Here's how the part is built. I have some questions about the finished solid (model axes, mm). Round coordinates to 2 decimals unless told otherwise and drop trailing zeros. Write each loop counter-clockwise with the first axis right and the second up, starting at its lowest first coordinate (ties: lowest second). Pieces come first, ordered by that corner, then holes. Notation, with made-up numbers: (-35, -33) -> (-3, -33) arc R21 cw to (-3, 1) -> close; hole circle Ø5 at (22, 30). An arc over 180 degrees is marked (long way). Answer in a Markdown table with one row per item.
from build123d import *

# Parameters (mm, degrees)
F0_W     = 457.2
F0_H     = 50.8
F1_DEPTH = 101.6
F2_W     = 98.554954
F2_H     = 50.8
F3_DEPTH = 2438.4
F4_W     = 457.2
F4_H     = 101.6
F5_DEPTH = 50.8


with BuildPart() as f1:
    # F0 (on Top) → F1 (new body)
    with BuildSketch(Plane.XY):
        with Locations((9.337193, 80.525405)):
            Rectangle(F0_W, F0_H)
        Polygon((-219.262807, 55.125405), (-219.262807, 105.925405), (-219.262807, 271.025405), (-270.062807, 271.025405), (-270.062807, -211.574595), (-219.262807, -211.574595), (-219.262807, -46.474595), (-219.262807, 4.325405), align=None)
        Polygon((237.937193, 271.025405), (237.937193, 105.925405), (237.937193, 55.125405), (237.937193, 4.325405), (237.937193, -46.474595), (237.937193, -211.574595), (288.737193, -211.574595), (288.737193, 271.025405), align=None)
        with Locations((9.337193, -21.074595)):
            Rectangle(F0_W, F0_H)
    extrude(amount=F1_DEPTH)

    # F2 (on Top) → F3 (join)
    with BuildSketch(Plane.XY):
        with Locations((-2.403777, 29.725405)):
            Rectangle(F2_W, F2_H)
    extrude(amount=F3_DEPTH)

    # F4 (on face) → F5 (join)
    with BuildSketch(Plane.XZ.offset(-4.325405)):
        with Locations((-2.403777, 2387.6)):
            Rectangle(F4_W, F4_H)
    extrude(amount=F5_DEPTH)


solid = f1.part
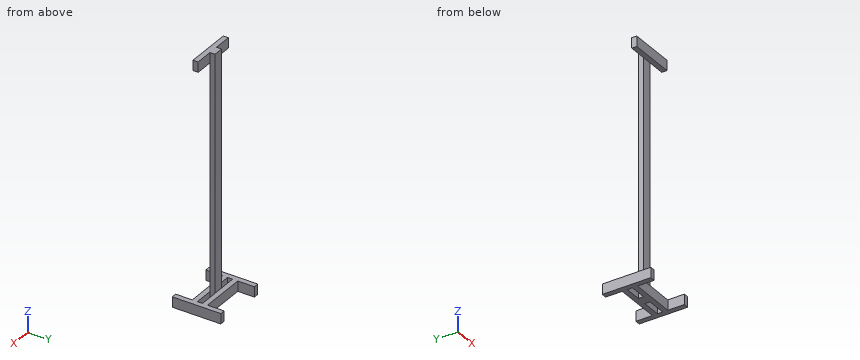
1) I need wall thicknesses on line 1 (Z direction, x = 136, y = -16.5); line 2 (Y direction, x = 199, z = 101); line 3 (Y direction, x = 31.5, z = 1650). Which ranges of each line are inside material? Lowest first, please. Write a range as [from, to].
Response:
| item | result |
|---|---|
| line 1 | z = [0, 101.6], [2336.8, 2438.4] |
| line 2 | y = [-46.47, 4.33], [55.13, 105.93] |
| line 3 | y = [4.33, 55.13] |
2) I want a section at B-B, the plane x = 126.5. List the corners of the cut face in (y, z) for me.
Response:
| item | result |
|---|---|
| outline | (-46.47, 0) -> (4.33, 0) -> (4.33, 101.6) -> (-46.47, 101.6) -> close; (-46.47, 2336.8) -> (4.33, 2336.8) -> (4.33, 2438.4) -> (-46.47, 2438.4) -> close; (55.13, 0) -> (105.93, 0) -> (105.93, 101.6) -> (55.13, 101.6) -> close |
3) I want a section at C-C, the plane z = 653. List the corners of the cut face in (x, y) for me, and give its area (3 significant figures).
Response:
| item | result |
|---|---|
| outline | (-51.68, 4.33) -> (46.87, 4.33) -> (46.87, 55.13) -> (-51.68, 55.13) -> close |
| area | 5,010 mm^2 |
4) I want a section at A-A, the plane y = 232.5. List the corners of the cut face in (x, z) for me.
Response:
| item | result |
|---|---|
| outline | (-270.06, 0) -> (-219.26, 0) -> (-219.26, 101.6) -> (-270.06, 101.6) -> close; (237.94, 0) -> (288.74, 0) -> (288.74, 101.6) -> (237.94, 101.6) -> close |
5) For pin 1 (1 mm diameter, centred on x = -180, y = 82, fed in from +Z); pin 2 (1.5 mm diameter, centred on x = 40.5, z = 2090.5, fed in from +Y); pin 3 (12 mm diameter, centred on x = -75.5, y = 44.5, fed in from -Z); pin 4 (15 mm diameter, centred on y = -20.5, z = 2403.5, fed in from +X), each with a flat end and sliding along its axis, tell me the tip position at first contact or that it passes through.
Response:
| item | result |
|---|---|
| pin 1 | stops at z = 101.6 |
| pin 2 | stops at y = 55.13 |
| pin 3 | passes through |
| pin 4 | stops at x = 226.2 |
